```python
from build123d import *

# Parameters (mm, degrees)
F0_R     = 1
F0_R_2   = 2.35
F1_DEPTH = 36
F2_W     = 275.678707
F2_H     = 30
F3_DEPTH = 26
F4_R     = 5


with BuildPart() as f1:
    # F0 (on Front) → F1 (new body)
    with BuildSketch(Plane.XZ):
        with BuildLine():
            Line((70, 5), (-10, 5))
            ThreePointArc((-10, 5), (-25, -10), (-10, -25))
            Line((-10, -25), (120, -25))
            Line((120, -25), (120, 5))
            Line((120, 5), (110, 5))
            Line((110, 5), (110, -15))
            Line((110, -15), (70, -15))
            Line((70, -15), (70, 5))
        make_face()
        with Locations((-10, -20)):
            Circle(F0_R, mode=Mode.SUBTRACT)
        with Locations((65.3, -11)):
            Circle(F0_R_2, mode=Mode.SUBTRACT)
        with Locations((114.7, -11)):
            Circle(F0_R_2, mode=Mode.SUBTRACT)
        with Locations((-20, -10)):
            Circle(F0_R, mode=Mode.SUBTRACT)
        with Locations((0, -10)):
            Circle(F0_R, mode=Mode.SUBTRACT)
        with Locations((-10, 0)):
            Circle(F0_R, mode=Mode.SUBTRACT)
        with Locations((65.3, 1)):
            Circle(F0_R_2, mode=Mode.SUBTRACT)
        with Locations((114.7, 1)):
            Circle(F0_R_2, mode=Mode.SUBTRACT)
    extrude(amount=F1_DEPTH)

    # F2 (on face) → F3 (cut)
    with BuildSketch(Plane.XZ.offset(36)):
        with Locations((-77.839354, -10)):
            Rectangle(F2_W, F2_H)
    extrude(amount=-F3_DEPTH, mode=Mode.SUBTRACT)

    # F4
    f4_edges = [f1.edges().sort_by_distance(p)[0] for p in [
        (110, -18, 5),
        (70, -18, 5),
    ]]
    fillet(f4_edges, radius=F4_R)


solid = f1.part
```
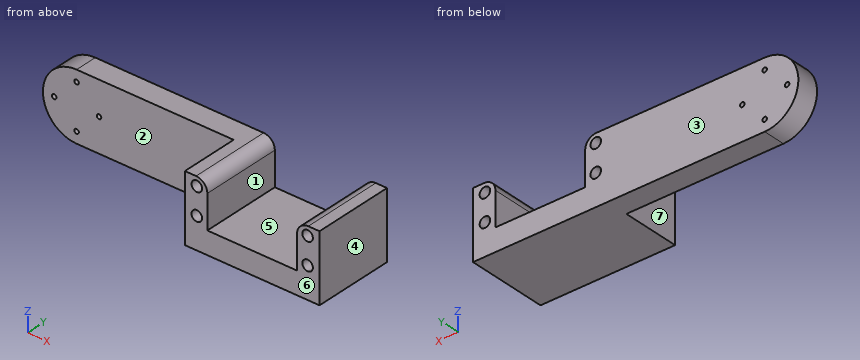
Geometry: final body of the model. Coordinates: model frame, mm. Face numbers are marked on the shaded views. A direction names the side the tool comes from. Round coordinates to 2 decimals unless told otherwise and drop trailing zeros. Order: outer loops, then holes, each group sorted by start corner. A loop starts at its lowest first (then second) coordinate and runs counter-clockwise, first axis right, second up. Notation, with made-up numbers: (22.5, 12) - (34.5, 12) arc R25 cw to (34.5, 32) - close; hole circle Ø7 at (84, 4.5). An arc over 180 degrees is marked (long way). Write item = value, one per line. Start each with the question number.
Q1. Cut plane B-B on y = -34. Return the cut outline in (x, z).
Q2. Cut plane D-D on x = 10. Return the cut outline in (y, z).
Q3. Access query for the marked faces 1, 2 and 3. Directions: +Z, -Z, +X, -X, +Y, -Y. A direction counts if a zero-diameter tool reaches every point of the face in a straight line with its end or side. Return the directions, or none.
Q4. Pin query (flat end, axial travel): pin 1 (7.5 mm diameter, centred on y = -17.5, z = -5.5, fed in from -X); pin 2 (3 mm diameter, centred on x = -10, z = -20, fed in from -Y); pin 3 (10 mm diameter, centred on x = 92, y = -9.5, fed in from +Z). Return the tip coordinate at first contact, or that it passes through.
Q5. Pull-direction query (X, two-part tool) for the marked faces 4, 5, 6 and 7; classes: +X half, -X half, draft (parallel to the pull), parting line (faces both ways), or undercut.
Q6. Ray query, line 1 (Z direction, x = -10, y = -5); line 2 (Z direction, x = 65, y = -15); line 3 (X direction, y = -7.75, z = -10). Return the intervals inside material, ascending. Write a range as from..to.
Q7. Cut plane A-A on y = -2.5. Give the number of separate pieces and of enclosed holes in the cut face, and give its area (3 significant figures).
Q8. Cut plane C-C on x = 73. Return the cut outline in (y, z).
Outcome:
q1.outline = (60, -25) - (120, -25) - (120, 5) - (115, 5) arc R5 ccw to (110, 0) - (110, -15) - (70, -15) - (70, 0) arc R5 ccw to (65, 5) - (60, 5) - close; hole circle Ø4.7 at (65.3, -11); hole circle Ø4.7 at (65.3, 1); hole circle Ø4.7 at (114.7, -11); hole circle Ø4.7 at (114.7, 1)
q2.outline = (-10, -25) - (0, -25) - (0, 5) - (-10, 5) - close
q3.face_1 = +Z, +Y, -Y
q3.face_2 = +Z, -Z, -X, -Y
q3.face_3 = +Z, -Z, +X, -X, +Y
q4.pin_1 = 60
q4.pin_2 = -10
q4.pin_3 = -15
q5.face_4 = +X half
q5.face_5 = undercut
q5.face_6 = draft
q5.face_7 = -X half
q6.line_1 = -25..-21, -19..-1, 1..5
q6.line_2 = -25..-13.33, -8.67..-1.33, 3.33..5
q6.line_3 = -25..-21, -19..-1, 1..63.17, 67.43..70, 110..112.57, 116.83..120
q7.separate_pieces = 1
q7.enclosed_holes = 8
q7.area = 3,360 mm^2
q8.outline = (-36, -25) - (0, -25) - (0, -15) - (-36, -15) - close
